Could you check a few things on this drawing? It's one solid part, dimensions in mm from its lowest x, y, z. A direction names the side the tool comes from. Give positions to 0.01 mm unless a question says otherwise; leave off trailing zeros. Loops run counter-clockwise (first coordinate to the right, second up) from the corner with the lowest first, then second, coordinate; pieces in that order, holes last. Notation, with made-up numbers: (-20, 28) - (16, 28) arc R19 cw to (16, 52) - close; hole circle Ø5 at (51, 27). An arc over 180 degrees is marked (long way). Return JSON: item names as keys, results as strings. Group by question number.
(1) If we section it at D-D (z = 28.5): Please give me the cut outline in (x, y) (1 decimal).
(2) For P1, Ø1.3, axis at x = 61, y = 1.5, coming from the +Z side; P2, Ø9, axis at y = 39.72, z = 24.94, coming from the +X side, each with a flat end and sliding along its axis, tell me the tip position at first contact or that it passes through.
(3) On a 3-axis mill with a long thin cutter (end or side, diameter ignored), from which of +Z, -Z, +X, -X, +Y, -Y can I reach the whole of each face in a straight line? I mean the marked faces 1 and 2. Say none if no direction works.
(4) If we mould it in two halves opening along X, with no side actions, what happens to the marked faces 3, 4 and 5? For each: released by +X, released by -X, zero draft, split by the parting line, or undercut.
(5) If we section it at C-C (y = 22): Please give me the cut outline in (x, z), then the cut area to 3 significant figures.
(6) I need wall thicknesses on probe 1 along Y at (x, z) = (66, 3); probe 2 along X at (y, z) = (11.5, 28.5). Which ranges of each line are inside material? Lowest first, please. Write a range as [from, to].
(7) If we section it at A-A (x = 40.5): Please give me the cut outline in (y, z).
(8) If we section it at B-B (z = 11): Please give me the cut outline in (x, y).
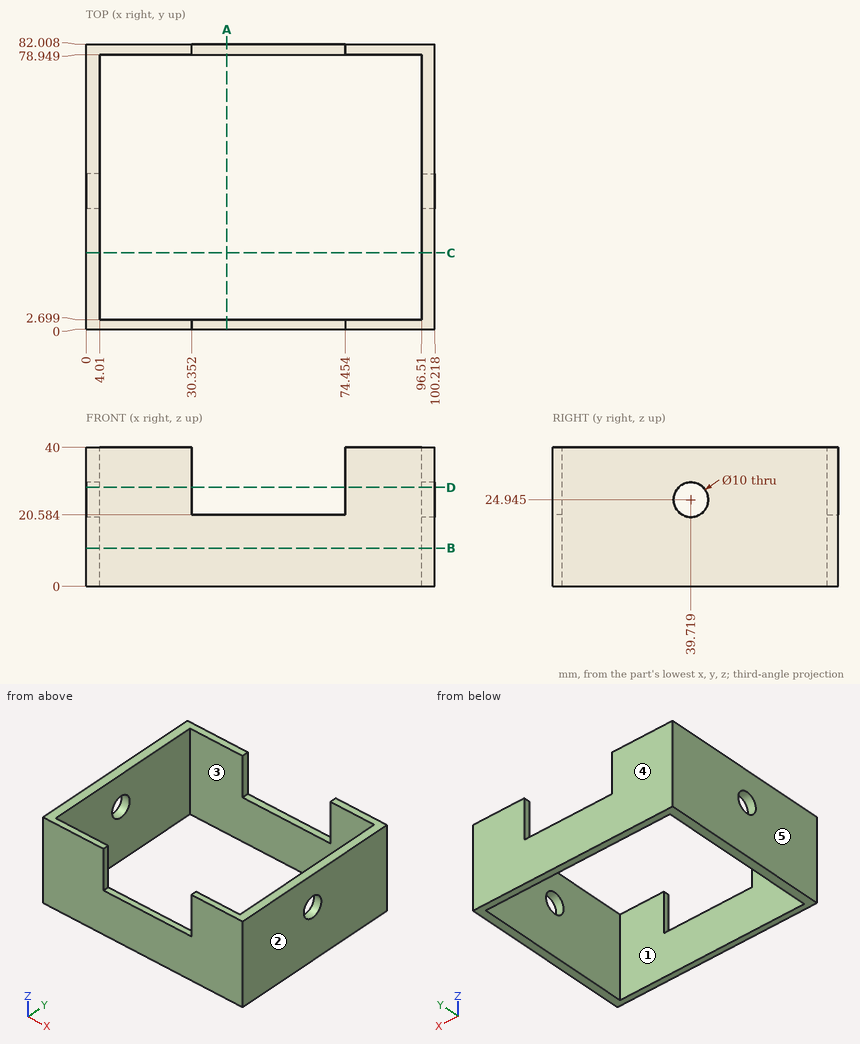
Values:
{
 "1": {"outline": "(0, 0) - (30.4, 0) - (30.4, 2.7) - (4, 2.7) - (4, 36.2) - (0, 36.2) - close; (0, 43.2) - (4, 43.2) - (4, 78.9) - (30.4, 78.9) - (30.4, 82) - (0, 82) - close; (74.5, 0) - (100.2, 0) - (100.2, 36.2) - (96.5, 36.2) - (96.5, 2.7) - (74.5, 2.7) - close; (74.5, 78.9) - (96.5, 78.9) - (96.5, 43.2) - (100.2, 43.2) - (100.2, 82) - (74.5, 82) - close"},
 "2": {"P1": "z = 20.58", "P2": "through"},
 "3": {"face 1": "+Z, -Z", "face 2": "+Z, -Z, +X, +Y, -Y"},
 "4": {"face 3": "undercut", "face 4": "zero draft", "face 5": "released by -X"},
 "5": {"outline": "(0, 0) - (4.01, 0) - (4.01, 40) - (0, 40) - close; (96.51, 0) - (100.22, 0) - (100.22, 40) - (96.51, 40) - close", "area": "309 mm2"},
 "6": {"probe 1": "[0, 2.7], [78.95, 82.01]", "probe 2": "[0, 4.01], [96.51, 100.22]"},
 "7": {"outline": "(0, 0) - (2.7, 0) - (2.7, 20.58) - (0, 20.58) - close; (78.95, 0) - (82.01, 0) - (82.01, 20.58) - (78.95, 20.58) - close"},
 "8": {"outline": "(0, 0) - (100.22, 0) - (100.22, 82.01) - (0, 82.01) - close; hole (4.01, 2.7) - (96.51, 2.7) - (96.51, 78.95) - (4.01, 78.95) - close"}
}
